Geometry: see drawing. Coordinates: mm, zero at the bounding-box minimum. Coordinates: 2 decimals unless noted, no trailing zeros. Write each loop counter-clockwise with the first axis right and the second up, starting at its lowest first coordinate (ties: lowest second). Pieces come first, ordered by that corner, then holes.
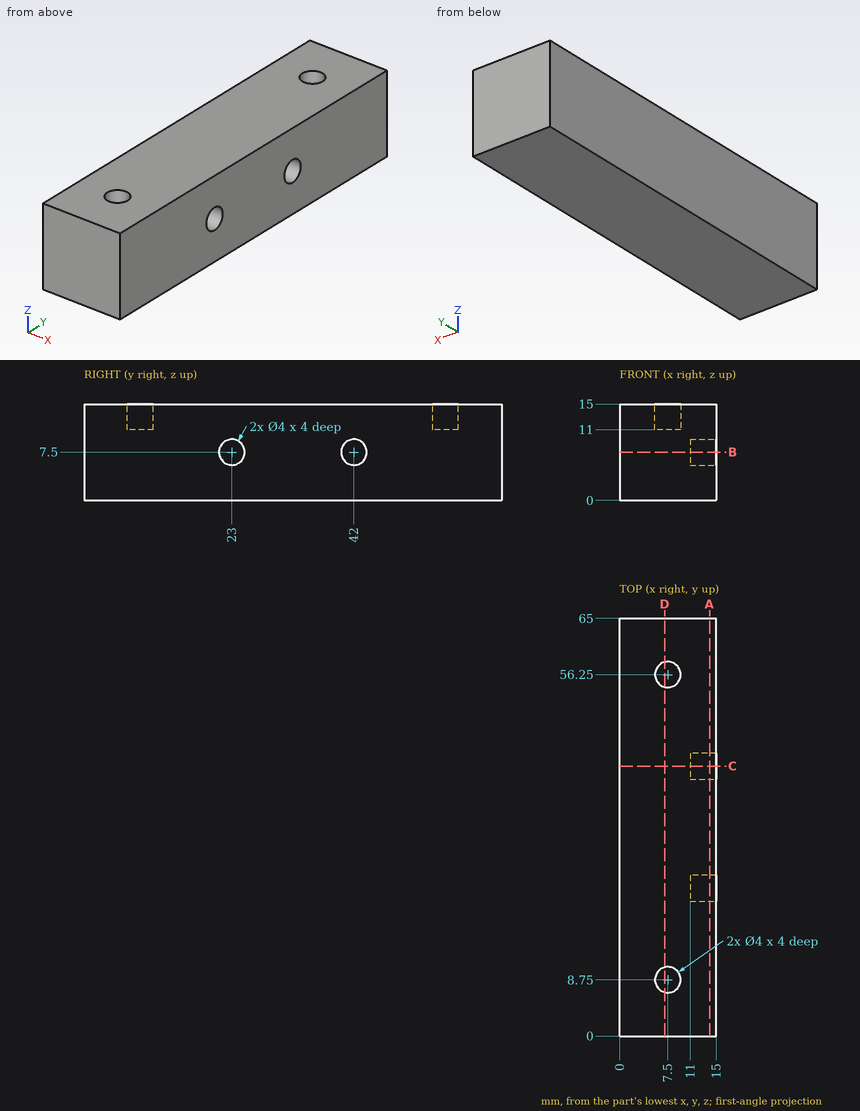
Item 1: Section D-D, the plane x = 7. Output: boundary loops of the cut face in (y, z).
Derived:
outline: (0, 0) - (65, 0) - (65, 15) - (58.19, 15) - (58.19, 11) - (54.31, 11) - (54.31, 15) - (10.69, 15) - (10.69, 11) - (6.81, 11) - (6.81, 15) - (0, 15) - close
Item 2: Material intervals for probe 1 along Y at (x, z) = (7.5, 13.9); probe 2 along Z at (x, y) = (12.95, 42), sorted ascending.
Derived:
probe 1: y = 0 to 6.75, 10.75 to 54.25, 58.25 to 65
probe 2: z = 0 to 5.5, 9.5 to 15
Item 3: Section B-B, the plane z = 7.5. Output: boundary loops of the cut face in (x, y), plus the area to 3 significant figures.
Derived:
outline: (0, 0) - (15, 0) - (15, 21) - (11, 21) - (11, 25) - (15, 25) - (15, 40) - (11, 40) - (11, 44) - (15, 44) - (15, 65) - (0, 65) - close
area: 943 mm2
Item 4: Section A-A, the plane x = 14. Output: boundary loops of the cut face in (y, z).
Derived:
outline: (0, 0) - (65, 0) - (65, 15) - (0, 15) - close; hole circle Ø4 at (23, 7.5); hole circle Ø4 at (42, 7.5)
Item 5: Pin query (flat end, axial travel): pin 1 (2.5 mm diameter, centred on x = 7.5, y = 8.75, fed in from +Z); pin 2 (2.5 mm diameter, centred on y = 42, z = 7.5, fed in from +X). Return the tip coordinate at first contact, or that it passes through.
Derived:
pin 1: stops at z = 11
pin 2: stops at x = 11
Item 6: Section C-C, the plane y = 42. Output: boundary loops of the cut face in (x, z).
Derived:
outline: (0, 0) - (15, 0) - (15, 5.5) - (11, 5.5) - (11, 9.5) - (15, 9.5) - (15, 15) - (0, 15) - close
